from build123d import *

# Parameters (mm, degrees)
F2_R     = 19.685
F2_R_2   = 3.175
F3_DEPTH = 9.525
F4_R     = 1.5875
F6_DEPTH = 5.207


with BuildPart() as f1:
    # F0 (on Front) → F1 (revolve)
    with BuildSketch(Plane.XZ):
        Polygon((-6.35, 38.1), (-6.35, 3.175), (6.35, 3.175), (6.35, 38.1), (5.588, 38.1), (3.175, 33.920561), (3.175, 22.86), (-3.175, 22.86), (-3.175, 33.920561), (-5.588, 38.1), align=None)
    revolve(axis=Axis((0, 0, 0), (1, 0, 0)))

    # F2 (on face) → F3 (cut)
    with BuildSketch(Plane(origin=(-6.35, 0, 0), x_dir=(0, -1, 0), z_dir=(-1, 0, 0))):
        Circle(F2_R)
        Circle(F2_R_2, mode=Mode.SUBTRACT)
    extrude(amount=-F3_DEPTH, mode=Mode.SUBTRACT)

    # F4
    f4_edges = [f1.edges().sort_by_distance(p)[0] for p in [
        (-6.35, 19.685, 0),
        (3.175, 19.685, 0),
        (-3.175, 0, -22.86),
        (3.175, 0, -22.86),
    ]]
    fillet(f4_edges, radius=F4_R)

    # F5 (on Right) → F6 (cut, symmetric)
    with BuildSketch(Plane.YZ):
        Polygon((-34.179726, 16.833192), (0, 22.86), (34.179726, 16.833192), (34.179726, 38.1), (-34.179726, 38.1), align=None)
    extrude(amount=F6_DEPTH, both=True, mode=Mode.SUBTRACT)


solid = f1.part
Could you check a few things on this model? Use its own coordinates, in mm. A direction names the side the tool comes from. Give positions to 0.01 mm unless a question says otherwise; leave off trailing zeros. Loops run counter-clockwise (first coordinate to the right, second up) from the corner with the lowest first, then second, coordinate; pieces in that order, holes last. Notation, with made-up numbers: (25.5, 51) -> (71.5, 51) arc R21 ccw to (71.5, 90) -> close; hole circle Ø8 at (39.25, -27). An arc over 180 degrees is marked (long way). Return JSON: item names as keys, results as strings.
Item 1: I'm going to push flat-ended pins straight in: pin 1 (18 mm diameter, centred on y = -2.5, z = 5, fed in from -X) (3 decimals); pin 2 (6 mm diameter, centred on x = 3.5, y = 25.5, fed in from -Z); pin 3 (1.5 mm diameter, centred on x = -2.5, y = -16.5, fed in from +Z). Where does each tip first touch, or does it pass through?
Geometry results:
{"pin 1": "stops at x = 3.175", "pin 2": "stops at z = -30.11", "pin 3": "stops at z = 20.01"}
Item 2: We'd pull the mould along Z, two halves only. Please class faces 4 (the cylindrical face through (-1.63, 15.62, -11.98)), 5 (the flat face through (3.175, 2, -25)), 6 (the flat face through (3.175, 0, -4)), 7 (the flat face through (3.544, 12.744, 20.613)): +Z half, -Z half, draft (parallel to the pull), parting line (faces both ways), or undercut.
Geometry results:
{"face 4": "undercut", "face 5": "draft", "face 6": "undercut", "face 7": "+Z half"}
Item 3: Which directions (+Z, -Z, +X, -X, +Y, -Y) give clear straight access to the entire face, cutting with the end or side of a thin tool? Please do faces 1 (the flat face through (3.54, -13.21, 20.53)), 2 (the conical face through (3.29, -1.5, -34.09)), 3 (the flat face through (-5.207, 0, 27)).
Geometry results:
{"face 1": "+Z, -Y", "face 2": "none", "face 3": "+Z"}
Item 4: If we section it at B-B on x = 0: List the corners of the cut face in (y, z) for me (3 decimals), plus the area to 3 significant figures.
Geometry results:
{"outline": "(-7.819, 21.481) arc R22.86 ccw (long way) to (7.819, 21.481) -> (0, 22.86) -> close; hole circle Ø39.37 at (0, 0)", "area": "421 mm²"}
Item 5: I need wall thicknesses on L1, parallel to Z at x = -1, y = 0 (3 decimals); L2, parallel to X at y = 28.5, z = 18; L3, parallel to X at y = 3.5, z = -29 (3 decimals). Which ranges of each line are inside material? Lowest first, please. Write a range as from..to.
Geometry results:
{"L1": "z = -22.86..-19.685, 19.685..22.86", "L2": "x = -6.35..-5.21, 5.21..6.35", "L3": "x = -6.35..-3.175, 3.175..6.35"}
